For this review, use the dimensioned drawing (mm, ordinates from the lowest corner) and the shaded views. A direction names the side the tool comes from. Round coordinates to 2 decimals unless told otherwise and drop trailing zeros. Write each loop counter-clockwise with the first axis right and the second up, starting at its lowest first coordinate (ties: lowest second). Pieces come first, ordered by that corner, then holes. Notation, with made-up numbers: (2, 54) -> (28, 54) arc R25 cw to (28, 91) -> close; hole circle Ø1 at (7, 54.25). An arc over 180 degrees is marked (long way). Answer as CSV lines item,"result". Start each with the question number.
Item 1: Mouldability with a two-part tool opening along X and no side actions: class the marked faces 3 and 4 as +X half, -X half, draft (parallel to the pull), parting line (faces both ways), or undercut.
Item 2: Take a section at B-B on z = 5. Give the boundary of the cut face in (x, y).
Item 3: Take a section at D-D on x = 10. Give the boundary of the cut face in (y, z), then the cut area to 3 significant figures.
Item 4: Machinability: for the marked faces 1 and 2, which of the approach directions +Z, -Z, +X, -X, +Y, -Y give a long, thin tool a straight path to every point of the face, cutting with its end or side? Answer none if there is none.
Item 5: Take a section at C-C on y = 1.1. Give the boundary of the cut face in (x, z), then the cut area to 3 significant figures.
Item 6: Take a section at A-A on x = 5.25. Give the boundary of the cut face in (y, z).
Item 7: Wall thickness on probe 1 along Z at (x, y) = (5, 1.05); probe 2 along X at (y, z) = (1.35, 3.5); probe 3 along Z at (x, y) = (10, 0.8): over which ranges is each line inside the solid? List them lowest first. Write a range as from..to.
Item 8: For pin 1 Ø0.8 at (y, z) = (1, 7) entering from -X, flat-tipped, find the tip position at first contact; note if it passes through.
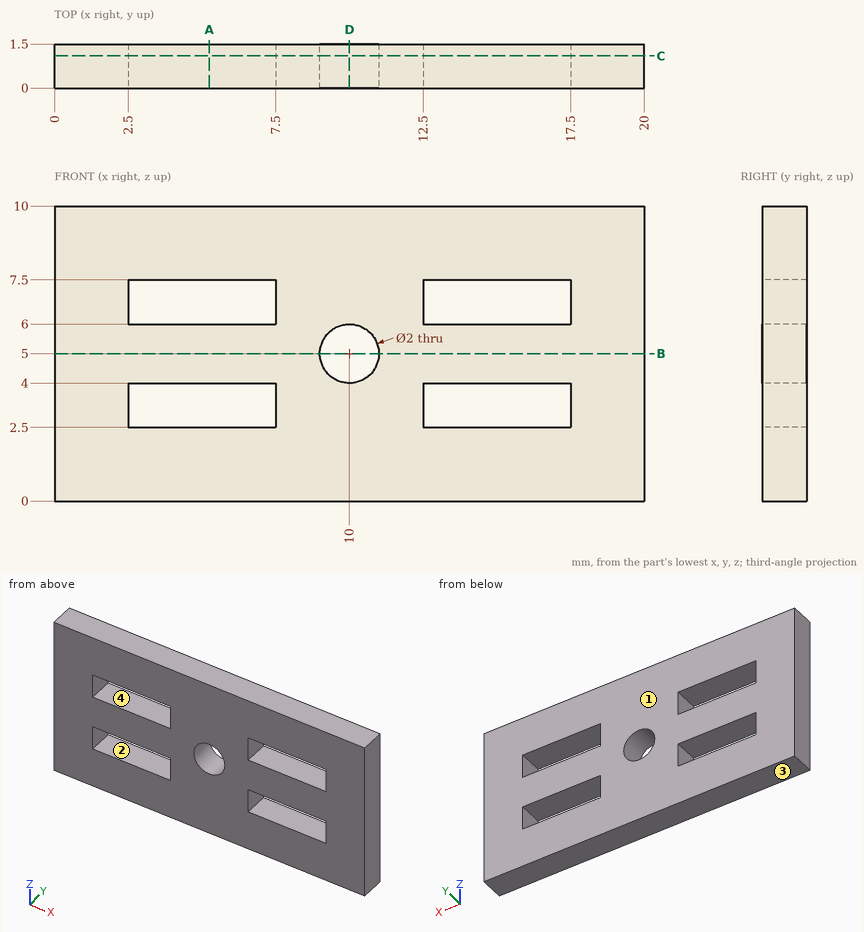
Output values:
1,face 3,"draft"
1,face 4,"undercut"
2,outline,"(0, 0) -> (9, 0) -> (9, 1.5) -> (0, 1.5) -> close; (11, 0) -> (20, 0) -> (20, 1.5) -> (11, 1.5) -> close"
3,outline,"(0, 0) -> (1.5, 0) -> (1.5, 4) -> (0, 4) -> close; (0, 6) -> (1.5, 6) -> (1.5, 10) -> (0, 10) -> close"
3,area,"12.0 mm^2"
4,face 1,"+Z, -Z, +X, -X, +Y"
4,face 2,"+Y, -Y"
5,outline,"(0, 0) -> (20, 0) -> (20, 10) -> (0, 10) -> close; hole (2.5, 2.5) -> (7.5, 2.5) -> (7.5, 4) -> (2.5, 4) -> close; hole (2.5, 6) -> (7.5, 6) -> (7.5, 7.5) -> (2.5, 7.5) -> close; hole circle Ø2 at (10, 5); hole (12.5, 2.5) -> (17.5, 2.5) -> (17.5, 4) -> (12.5, 4) -> close; hole (12.5, 6) -> (17.5, 6) -> (17.5, 7.5) -> (12.5, 7.5) -> close"
5,area,"167 mm^2"
6,outline,"(0, 0) -> (1.5, 0) -> (1.5, 2.5) -> (0, 2.5) -> close; (0, 4) -> (1.5, 4) -> (1.5, 6) -> (0, 6) -> close; (0, 7.5) -> (1.5, 7.5) -> (1.5, 10) -> (0, 10) -> close"
7,probe 1,"z = 0..2.5, 4..6, 7.5..10"
7,probe 2,"x = 0..2.5, 7.5..12.5, 17.5..20"
7,probe 3,"z = 0..4, 6..10"
8,pin 1,"stops at x = 0"
